Geometry: final body of the model. Coordinates: model frame, mm. A direction names the side the tool comes from. Round coordinates to 2 decimals unless told otherwise and drop trailing zeros. Write each loop counter-clockwise with the first axis right and the second up, starting at its lowest first coordinate (ties: lowest second). Pieces come first, ordered by that corner, then holes.
Autodesk Inventor part; units mm, degrees
ref_plane "Work Plane1" through (0, 0, 2) normal (0, 0, 1) x (1, 0, 0)
ref_plane "Work Plane2" through (0, 0, 2) normal (0, 0, -1) x (-1, 0, 0)
ref_plane "YZ Plane" through (0, 0, 0) normal (1, 0, 0) x (0, 1, 0)
sketch "Sketch1" plane through (0, 0, 0) normal (0, 0, 1) x (1, 0, 0)
  circle A0 centre (0, 0) radius 1
  circle A1 centre (0, 0) radius 2.25
  circle A2 centre (0, 40) radius 1
  circle A3 centre (0, 40) radius 2.25
  line L0 (-2.25, 40) -> (-2.25, 0)
  line L1 (0, 0) -> (15, 0) construction
  line L2 (12.2873, 8.6036) -> (11.2873, 8.6036)
  circle A4 centre (12.2873, 8.6036) radius 1
  circle A5 centre (12.2873, 8.6036) radius 2.25
  line L3 (2.25, 0) -> (13.4395, 6.671)
  line L4 (2.25, 40) -> (7.9069, 34.3431)
  line L5 (7.9069, 34.3431) -> (7.9069, 19.3431)
  line L6 (7.9069, 19.3431) -> (14.1662, 9.8414)
  line L7 (0, 0) -> (0, 1)
  line L8 (0, 39) -> (0, 40)
  line L9 (0, 0) -> (1.8431, 1.2905)
  line L10 (11.4681, 8.0301) -> (12.2873, 8.6036)
  dimension "d5" = 2
  dimension "d7" = 2
  dimension "d0" = 40
  dimension "d6" = 4.5
  dimension "d8" = 4.5
  dimension "d9" = 15
  dimension "d11" = 2
  dimension "d12" = 4.5
  dimension "d13" = 8
  dimension "d15" = 15
ref_plane "Work Plane1" through (0, 0, 2) normal (0, 0, 1) x (1, 0, 0)
extrude "Extrusion1" add sketch "Sketch1" against normal blind 2.5 contours A1 L0 A3 L4 L5 L6 A5 L3
extrude "Extrusion2" add sketch "Sketch1" against normal blind 2 contours A1 | A5 | A3
mirror "Mirror1" about plane through (0, 0, 2) normal (0, 0, 1) of "Extrusion1", "Extrusion2"
sketch "Sketch2" plane through (0, 0, 0) normal (0, 0, 1) x (1, 0, 0)
  line L0 (0, 37.5855) -> (-2.2556, 37.5855)
  line L1 (-2.2556, 37.5855) -> (-2.2556, 29.5855)
  line L2 (-2.2556, 29.5855) -> (0, 29.5855)
  line L3 (0, 29.5855) -> (0, 37.5855)
  point P0 (0, 0)
  dimension "d21" = 8
extrude "Extrusion3" add sketch "Sketch2" along normal blind 6
sketch "Sketch3" plane through (0, 0, 6.5) normal (0, 0, 1) x (1, 0, 0)
  line L0 (7.9069, 19.3431) -> (5.9069, 19.3431)
  line L1 (5.9069, 19.3431) -> (5.9069, 27.3431)
  line L2 (5.9069, 27.3431) -> (7.9069, 27.3431)
  line L3 (7.9069, 27.3431) -> (7.9069, 19.3431)
  point P0 (0, 0)
  dimension "d24" = 2
  dimension "d25" = 8
extrude "Extrusion4" add sketch "Sketch3" against normal blind 9
sketch "Sketch6" plane through (0, 0, 4) normal (0, 0, -1) x (-1, 0, 0)
  circle A0 centre (0, 0) radius 4.5
  dimension "d33" = 9
extrude "Extrusion7" cut sketch "Sketch6" against normal blind 0.5
sketch "Sketch7" plane through (0, 0, 0) normal (0, 0, 1) x (1, 0, 0)
  circle A0 centre (0, 0) radius 4.5
  dimension "d36" = 9
extrude "Extrusion8" cut sketch "Sketch7" against normal blind 0.5
sketch "Sketch8" plane through (0, 40, 4) normal (0, 0, -1) x (-1, 0, 0)
  circle A0 centre (0, 0) radius 2.5
  circle A1 centre (0, 0) radius 2.5
  line L0 (-7.9069, -5.6569) -> (-2.4944, -0.2556)
  arc A2 (-2.4876, -0.2488) -> (-1.7678, -1.7678) centre (0, 0) ccw
  arc A3 (-2.4876, -0.2488) -> (-1.7678, -1.7678) centre (0, 0) ccw
  line L1 (-7.9069, -5.6569) -> (-2.4876, -0.2488)
  line L2 (-7.9069, -5.6569) -> (-7.9069, -7.9069)
  line L3 (1.2823, -2.1461) -> (-7.9069, -11.3352)
  line L4 (-7.9069, -12.6569) -> (-7.9069, -5.6569)
  point P0 (0, -40)
  dimension "d39" = 5
extrude "Extrusion9" cut sketch "Sketch8" against normal blind 0.5
ref_plane "Work Plane2" through (0, 0, 2) normal (0, 0, -1) x (-1, 0, 0)
mirror "Mirror2" about plane through (0, 0, 2) normal (0, 0, -1) of "Extrusion9"
extrude "Extrusion10" cut sketch "Sketch8" along normal blind 0.5 contours A0 L3 L4 L2 L0 L1
mirror "Mirror3" about plane through (0, 0, 2) normal (0, 0, -1) of "Extrusion9"
properties part number "Pinky_Lower_main_1"
1) Section C-C on z = -1. Output: boundary loops of the cut face in (x, y), plus the area to 3 significant figures.
2) Section D-D on y = 23.5. Output: boundary loops of the cut face in (x, z), plus the area to 3 significant figures.
3) Section B-B on x = 9.5. Output: boundary loops of the cut face in (y, z).
4) First-contact query: P1, Ø3, axis at y = 5.5, z = 0.5, coming from the -X side; P2, Ø3.5, axis at x = 13, y = 7.5, coming from the -Z side; P3, Ø5, axis at x = 8.5, z = -1, coming from the -Y side; P4, Ø2.5, axis at x = 12.29, y = 8.6, coming from the +Z side. Flat tips, straight axial feed; report the tip coordinate or a pass-through.
5) Draft query along Z for faces 5 (the cylindrical face through (10.112, 9.178, -2.246)), 6 (the flat face through (0, 34, 2)), 7 (the flat face through (4, 20, -2.5)). Return one class per face: pulls with the +Z half, pulls with the -Z half, needs draft (parallel to the pull), parting line crosses it, or undercut.
6) Section A-A on y = 14. Output: boundary loops of the cut face in (x, z), plus the area to 3 significant figures.
7) Line query: probe 1 along Y at (x, z) = (0, -1.45); probe 2 along Z at (x, y) = (-1.25, 24); probe 3 along Z at (x, y) = (1.75, 0). Output: solid intervals per line, ascending.
8) Reachability of faces 1 (the cylindrical face through (-0.05, 37.75, -2.25)), 2 (the flat face through (3, 36, -0.5)), 3 (the cylindrical face through (0.05, 2.25, -2.25)), 4 (the flat face through (-2, 38, 4)) from +Z, -Z, +X, -X, +Y, -Y: full face, straight path, thin tool, end or side. Return the list, or none.
Filled in:
1. outline: (-2.25, 0) arc R2.25 ccw to (2.25, 0) - (13.44, 6.67) arc R2.25 ccw to (14.17, 9.84) - (7.91, 19.34) - (7.91, 34.34) - (2.25, 40) arc R2.25 ccw to (-2.25, 40) - close; hole circle Ø2 at (0, 0); hole circle Ø2 at (0, 40); hole circle Ø2 at (12.29, 8.6)
1. area: 446 mm2
2. outline: (-2.25, -2.5) - (7.91, -2.5) - (7.91, 6.5) - (-2.25, 6.5) - (-2.25, 4) - (5.91, 4) - (5.91, 0) - (-2.25, 0) - close
2. area: 58.8 mm2
3. outline: (4.32, -2.5) - (16.92, -2.5) - (16.92, 0) - (4.32, 0) - close; (4.32, 4) - (16.92, 4) - (16.92, 6.5) - (4.32, 6.5) - close
4. P1: stops at x = -2.25
4. P2: stops at z = -2.5
4. P3: stops at y = 2.24
4. P4: stops at z = 6
5. face 5: needs draft
5. face 6: undercut
5. face 7: pulls with the -Z half
6. outline: (-2.25, -2.5) - (11.43, -2.5) - (11.43, 0) - (-2.25, 0) - close; (-2.25, 4) - (11.43, 4) - (11.43, 6.5) - (-2.25, 6.5) - close
6. area: 68.4 mm2
7. probe 1: y = -2.25 to -1, 1 to 39, 41 to 42.25
7. probe 2: z = -2.5 to 0, 4 to 6.5
7. probe 3: z = -2 to -0.5, 4.5 to 6
8. face 1: -Z, +Y
8. face 2: none
8. face 3: -Z, -Y
8. face 4: +X, -X, +Y
